Check sheet for the modelled part. Datum: model origin and axes. Units: mm. A direction names the side the tool comes from. Round coordinates to 2 decimals unless told otherwise and drop trailing zeros. Write each loop counter-clockwise with the first axis right and the second up, starting at its lowest first coordinate (ties: lowest second). Pieces come first, ordered by that corner, then holes. Notation, with made-up numbers: M 74,65.5 L 100,65.5 A17 ccw 100,81.5 Z; hole C 29.25,13 d4. An arc over 180 degrees is marked long. One line per item, written item: value.
from build123d import *

# Parameters (mm, degrees)
SKETCH1_R           = 3
BOSS_EXTRUDE1_DEPTH = 1.6
BOSS_EXTRUDE3_START = 4.5
BOSS_EXTRUDE3_DEPTH = 4.5


with BuildPart() as part:
    # Sketch1 → Boss-Extrude1 (new body)
    with BuildSketch(Plane(origin=(0, 0, 0), x_dir=(1, 0, 0), z_dir=(0, 1, 0))):
        with BuildLine():
            Line((1.268248439, -7.422428571), (-1.268248439, -7.422428571))
            ThreePointArc((-1.268248439, -7.422428571), (-4.955504601, -5.669556786), (-7.185986362, -2.25))
            Line((-7.185986362, -2.25), (-7.185986362, 2.25))
            ThreePointArc((-7.185986362, 2.25), (-4.955504601, 5.669556786), (-1.268248439, 7.422428571))
            Line((-1.268248439, 7.422428571), (1.268248439, 7.422428571))
            ThreePointArc((1.268248439, 7.422428571), (4.955504601, 5.669556786), (7.185986362, 2.25))
            Line((7.185986362, 2.25), (7.185986362, -2.25))
            ThreePointArc((7.185986362, -2.25), (4.955504601, -5.669556786), (1.268248439, -7.422428571))
        make_face()
        with Locations(Location((0, 0, 0), (0, 0, 270))):
            Circle(SKETCH1_R, mode=Mode.SUBTRACT)
    extrude(amount=BOSS_EXTRUDE1_DEPTH)

    # Sketch2 → Boss-Extrude3 (add)
    with BuildSketch(Plane.XZ.offset(BOSS_EXTRUDE3_START)):
        with BuildLine():
            ThreePointArc((-7.185986362, -2.25), (-6.924787857, -2.957737841), (-6.594083964, -3.635788316))
            Line((-6.594083964, -3.635788316), (-6.185986362, -3.635788316))
            Line((-6.185986362, -3.635788316), (-6.185986362, 3.764211684))
            Line((-6.185986362, 3.764211684), (-6.521626362, 3.764211684))
            ThreePointArc((-6.521626362, 3.764211684), (-6.895496422, 3.025397345), (-7.185986362, 2.25))
            Line((-7.185986362, 2.25), (-7.185986362, -2.25))
        make_face()
        with BuildLine():
            Line((6.185986362, -3.620011298), (6.602758378, -3.620011298))
            ThreePointArc((6.602758378, -3.620011298), (6.928318925, -2.949457048), (7.185986362, -2.25))
            Line((7.185986362, -2.25), (7.185986362, 2.25))
            ThreePointArc((7.185986362, 2.25), (6.891829312, 3.033741706), (6.512494562, 3.779988702))
            Line((6.512494562, 3.779988702), (6.185986362, 3.779988702))
            Line((6.185986362, 3.779988702), (6.185986362, -3.620011298))
        make_face()
    extrude(amount=-BOSS_EXTRUDE3_DEPTH)


solid = part.part
Q1. Sectioned sample at C-C on y = -0.5. Enter the section's corners in (x, z).
Completed:
outline: M -7.19,-2.25 A7.53 ccw -6.59,-3.64 L -6.19,-3.64 L -6.19,3.76 L -6.52,3.76 A7.53 ccw -7.19,2.25 Z; M 6.19,-3.62 L 6.6,-3.62 A7.53 ccw 7.19,-2.25 L 7.19,2.25 A7.53 ccw 6.51,3.78 L 6.19,3.78 Z
Q2. Depth check by flat-ended pin: P1, Ø2, axis at x = -5.5, z = -1, coming from the -Y side; P2, Ø3, axis at y = 0, z = -5, coming from the +X side; P3, Ø3, axis at x = 1.5, z = 5, coming from the -Y side. Enter the tip coordinate at first touch or a pass-through.
Completed:
P1: y = -4.5
P2: x = 6.67
P3: y = 0
Q3. Scan lines: line 1 (X direction, y = -1.25, z = 1.75); line 2 (X direction, y = 1.25, z = 0); line 3 (Y direction, x = 2, z = 3.5). Record each from-to range of solid material in increasing order. Write a range as [from, to].
Completed:
line 1: [-7.19, -6.19], [6.19, 7.19]
line 2: [-7.19, -3], [3, 7.19]
line 3: [0, 1.6]
Q4. Sectioned sample at D-D on z = 5.25. Enter the section's corners in (x, y).
Completed:
outline: M -5.4,0 L 5.4,0 L 5.4,1.6 L -5.4,1.6 Z
Q5. Sectioned sample at A-A on z = 0. Enter the section's corners in (x, y).
Completed:
outline: M -7.19,-4.5 L -6.19,-4.5 L -6.19,0 L -3,0 L -3,1.6 L -7.19,1.6 Z; M 3,0 L 6.19,0 L 6.19,-4.5 L 7.19,-4.5 L 7.19,1.6 L 3,1.6 Z
Q6. Sectioned sample at B-B on x = 0. Enter the section's corners in (y, z).
Completed:
outline: M 0,-7.42 L 1.6,-7.42 L 1.6,-3 L 0,-3 Z; M 0,3 L 1.6,3 L 1.6,7.42 L 0,7.42 Z
Q7. Access from +Z, -Z, +X, -X, +Y, -Y to the whole of each face (thin tool, end or side, straight path). Record for faces 1 (the flat face through (6.186, -2, 0)), 2 (the flat face through (-7.186, -1, 0)).
Completed:
face 1: +Z, -Z, -Y
face 2: +Z, -Z, -X, +Y, -Y
Q8. Draft check along Z on faces 3 (the flat face through (0, 1, -7.422)), 4 (the cylindrical face through (0.9, 0.79, 2.86)), 5 (the flat face through (3.3, 1.6, -0.1)), 6 (the flat face through (0, 1, 7.422)). Enter one of: pulls with the +Z half, pulls with the -Z half, needs draft (parallel to the pull), parting line crosses it, or undercut.
Completed:
face 3: pulls with the -Z half
face 4: undercut
face 5: needs draft
face 6: pulls with the +Z half
